The model under review builds one solid part; all positions refer to its coordinate system, in mm. Face numbers are marked on the shaded views. Coordinates: 2 decimals unless noted, no trailing zeros. Write each loop counter-clockwise with the first axis right and the second up, starting at its lowest first coordinate (ties: lowest second). Pieces come first, ordered by that corner, then holes. Notation, with made-up numbers: (-6.5, 42.25) -> (3.5, 42.25) arc R19 cw to (3.5, 49.25) -> close; hole circle Ø4 at (58.25, 26). An arc over 180 degrees is marked (long way). Put each result on its own line as item: value. Start each with the question number.
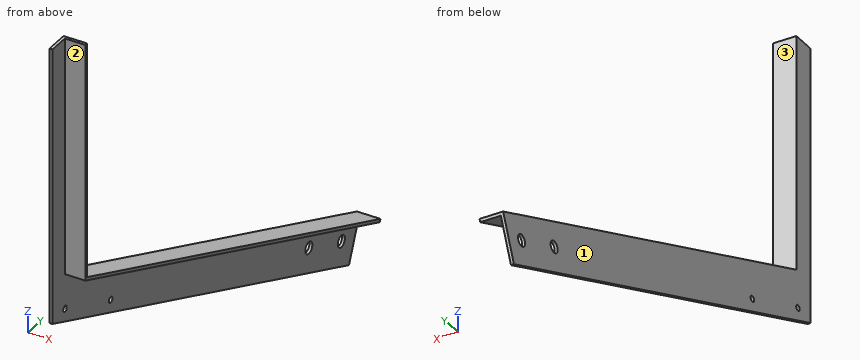
Autodesk Inventor part; units mm, degrees
ref_plane "YZ Plane" through (0, 0, 0) normal (1, 0, 0) x (0, 1, 0)
ref_plane "XZ Plane" through (0, 0, 0) normal (0, 1, 0) x (-1, 0, 0)
ref_plane "XY Plane" through (0, 0, 0) normal (0, 0, 1) x (1, 0, 0)
sketch "Sketch1" plane through (0, 0, 0) normal (1, 0, 0) x (0, 1, 0)
  line L0 (0, 0) -> (0, 254)
  line L1 (0, 0) -> (254, 0) construction
  line L2 (0, 0) -> (527.9972, -218.7036)
  line L3 (0, 0) -> (571.5, 0) construction
  line L4 (0, 254) -> (-25.4, 254)
  line L5 (0, 254) -> (25.4, 254) construction
  line L6 (527.9972, -218.7036) -> (508.5568, -265.6367)
  line L7 (527.9972, -218.7036) -> (578.7972, -218.7036) construction
  line L8 (508.5568, -265.6367) -> (-19.4403, -46.9331)
  line L9 (-19.4403, -46.9331) -> (-6.7403, -46.9331) construction
  line L10 (-25.4, 254) -> (-25.4, -44.4645)
  line L11 (-25.4, 254) -> (273.0645, 254) construction
  line L12 (-25.4, -44.4645) -> (-19.4403, -46.9331)
  line L13 (518.277, -242.1701) -> (543.677, -242.1701) construction
  circle A0 centre (494.8105, -232.45) radius 6.35
  circle A1 centre (436.1441, -208.1496) radius 6.35
  line L14 (-19.4403, -46.9331) -> (-14.5802, -35.1998)
  line L15 (126.219, -93.5208) -> (121.3589, -105.254)
  line L16 (-14.5802, -35.1998) -> (-1.8802, -35.1998) construction
  line L17 (-2.847, -40.0599) -> (86.053, -40.0599) construction
  circle A2 centre (79.2859, -74.0804) radius 3.175
  circle A3 centre (-2.847, -40.0599) radius 3.175
  dimension "d0" = 254
  dimension "d1" = 90
  dimension "d2" = 571.5
  dimension "d3" = 22.5
  dimension "d4" = 25.4
  dimension "d5" = 180
  dimension "d6" = 50.8
  dimension "d7" = 112.5
  dimension "d8" = 571.5
  dimension "d9" = 90
  dimension "d12" = 90
  dimension "d17" = 12.7
  dimension "d18" = 12.7
  dimension "d19" = 12.7
  dimension "d20" = 152.4
  dimension "d22" = 12.7
  dimension "d26" = 6.35
  dimension "d27" = 6.35
extrude "Extrusion1" add sketch "Sketch1" along normal blind 3.175
sketch "Sketch2" plane through (3.175, 0, 0) normal (1, 0, 0) x (0, 0, -1)
  line L0 (0, 0) -> (-254, 0)
  line L1 (265.6367, 508.5568) -> (218.7036, 527.9972)
  line L2 (218.7036, 527.9972) -> (0, 0)
  line L3 (218.7036, 527.9972) -> (221.6369, 526.7821)
  line L4 (218.7036, 527.9972) -> (221.8786, 527.9972) construction
  line L5 (-254, 0) -> (-254, -3.175)
  line L6 (-254, 0) -> (-250.825, 0) construction
  line L7 (-254, -3.175) -> (2.1215, -3.175)
  line L8 (2.1215, -3.175) -> (221.6369, 526.7821)
  dimension "d30" = 3.175
  dimension "d31" = 22.5
  dimension "d33" = 3.175
  dimension "d34" = 90
  dimension "d35" = 90
extrude "Extrusion2" add sketch "Sketch2" along normal blind 22.225
properties part number "CatapultArmZ-Left"
1. Consider section C-C on x = 8.5. State the section outline as (y, z) points (1 decimal), then the cut area to 3 significant figures.
2. Insertion check: P1, Ø5, axis at y = 354.5, z = -177.5, coming from the +X side (3 decimals); P2, Ø12, axis at x = 14.5, y = 133, coming from the +Z side; P3, Ø1, axis at x = 7, z = 117, coming from the -Y side (3 decimals); P4, Ø7.5, axis at y = 494.81, z = -232.45, coming from the +X side. Each pin has a flat end and moves straight along its axis. Give the tip position at first contact, or say it passes through.
3. Wall thickness on line 1 (X direction, y = 79, z = -63) (3 decimals); line 2 (Y direction, x = 5.25, z = 79) (3 decimals); line 3 (Y direction, x = 2.75, z = 133.5): over which ranges is each line inside the solid? List them lowest first. Write a range as from..to.
4. Consider section B-B on z = -232.45. State the section outline as (x, y) points (1 decimal).
5. The part is to be moulded in two halves that separate along Y. For the marked faces 1, 2 and 3, say which applies: released by +Y, released by -Y, zero draft, split by the parting line, or undercut.
6. Consider section A-A on z = 20. State the section outline as (x, y) points (3 decimals).
Output values:
1. outline: (-3.2, -2.1) -> (526.8, -221.6) -> (528, -218.7) -> (0, 0) -> (0, 254) -> (-3.2, 254) -> close
1. area: 2,630 mm^2
2. P1: stops at x = 3.175
2. P2: stops at z = -52.61
2. P3: stops at y = -3.175
2. P4: passes through
3. line 1: x = 0..3.175
3. line 2: y = -3.175..0
3. line 3: y = -25.4..0
4. outline: (0, 428.4) -> (3.2, 428.4) -> (3.2, 488.5) -> (0, 488.5) -> close; (0, 501.2) -> (3.2, 501.2) -> (3.2, 522.3) -> (0, 522.3) -> close
5. face 1: zero draft
5. face 2: released by -Y
5. face 3: released by +Y
6. outline: (0, -25.4) -> (3.175, -25.4) -> (3.175, -3.175) -> (25.4, -3.175) -> (25.4, 0) -> (0, 0) -> close
